from build123d import *

# Parameters (mm, degrees)
BOSS_EXTRUDE1_DEPTH = 300
SKETCH3_R           = 1.6
CUT_EXTRUDE1_DEPTH  = 331.850051567
CUT_EXTRUDE2_START  = -2
SKETCH4_R           = 2.875
CUT_EXTRUDE2_DEPTH  = 329.850051657


with BuildPart() as part:
    # Sketch2 → Boss-Extrude1 (new body)
    with BuildSketch(Plane.XY):
        with BuildLine():
            Line((-10, 0), (-10, 57.592991829))
            Line((-10, 57.592991829), (-14, 57.592991829))
            Line((-14, 57.592991829), (-14, 59.592991829))
            Line((-14, 59.592991829), (-10, 59.592991829))
            Line((-10, 59.592991829), (-5, 59.592991829))
            Line((-5, 59.592991829), (-5, 0))
            ThreePointArc((-5, 0), (-3.13691529, -11.76748288), (2.270101024, -22.383928263))
            Line((2.270101024, -22.383928263), (29.120915128, -37.886253013))
            ThreePointArc((29.120915128, -37.886253013), (41.018534684, -37.260643809), (52.141016151, -32.990381057))
            Line((52.141016151, -32.990381057), (103.750060963, -3.193885142))
            Line((103.750060963, -3.193885142), (106.250060963, -7.524012161))
            Line((106.250060963, -7.524012161), (108.250060963, -10.988113776))
            Line((108.250060963, -10.988113776), (106.518010155, -11.988113776))
            Line((106.518010155, -11.988113776), (104.518010155, -8.524012161))
            Line((104.518010155, -8.524012161), (54.641016151, -37.320508076))
            ThreePointArc((54.641016151, -37.320508076), (11.547005384, -37.320508076), (-10, 0))
        make_face()
    extrude(amount=BOSS_EXTRUDE1_DEPTH)

    # Sketch3 → Cut-Extrude1 (cut, through all)
    with BuildSketch(Plane(origin=(-9.125, -15.804963619, 0), x_dir=(0.8660254037844395, -0.49999999999999856, 0), z_dir=(0.49999999999999856, 0.8660254037844395, 0))):
        with Locations(Location((28.660254038, -15, 0), (0, 0, 180))):
            Circle(SKETCH3_R)
        with Locations(Location((28.660254038, -285, 0), (0, 0, 180))):
            Circle(SKETCH3_R)
    extrude(amount=-CUT_EXTRUDE1_DEPTH, mode=Mode.SUBTRACT)

    # Sketch4 → Cut-Extrude2 (cut, through all)
    with BuildSketch(Plane(origin=(-9.125, -15.804963619, 0), x_dir=(0.8660254037844395, -0.49999999999999856, 0), z_dir=(0.49999999999999856, 0.8660254037844395, 0)).offset(CUT_EXTRUDE2_START)):
        with Locations(Location((28.660254038, -15, 0), (0, 0, 180))):
            Circle(SKETCH4_R)
        with Locations(Location((28.660254038, -285, 0), (0, 0, 180))):
            Circle(SKETCH4_R)
    extrude(amount=-CUT_EXTRUDE2_DEPTH, mode=Mode.SUBTRACT)


solid = part.part
Geometry check sheet. Reference: the model listing, model coordinates, mm. A direction names the side the tool comes from. Coordinates: 2 decimals unless noted, no trailing zeros. Loops run counter-clockwise (first coordinate to the right, second up) from the corner with the lowest first, then second, coordinate; pieces in that order, holes last. Notation, with made-up numbers: (60, -26) - (105, -26) arc R18 ccw to (105, -3) - close; hole circle Ø2 at (20.25, -17.75). An arc over 180 degrees is marked (long way). Use one line per item in the form item = value. Start each with the question number.
Item 1: Tool access check on faces 1 (the face through (13.47, -34.74, 287.85)), 2 (the face through (15.51, -30.03, 147.9)), 3 (the face through (-10, 28, 148)). Record the directions out of +Z, -Z, +X, -X, +Y, -Y that give a thin tool (end or side, any length) a straight path to the whole face; none if there is none.
Item 2: Thickness scan on probe 1 along Y at (x, z) = (31, 179); probe 2 along X at (y, z) = (-2, 182); probe 3 along X at (y, z) = (-16.5, 276.5). Record the ranges inside material, lowest first.
Item 3: Section check B-B, the plane y = 5. Enter the section's corners in (x, z).
Item 4: Gauge pin test, flat ends, axial feed: pin 1 (1 mm diameter, centred on y = 36.5, z = 207.5, fed in from -X); pin 2 (10 mm diameter, centred on y = -21, z = 111.5, fed in from +X); pin 3 (1.5 mm diameter, centred on x = 5, z = 259.5, fed in from +Y). Record the tip position at first contact, or that the pin passes through.
Item 5: Section check C-C, the plane x = 34. Enter the section's corners in (y, z), and give its area (3 significant figures).
Item 6: Section check A-A, the plane z = 25. Enter the section's corners in (x, y).
Item 7: Mould release check, pull along X, two halves, no side actions. Record for faces 4 (the face through (-3.188, -11.608, 147.9)), 5 (the face through (12.096, -37.632, 147.9)), 6 (the face through (-5, 30, 148)), 7 (the face through (20, -33, 0)): +X half, -X half, draft (parallel to the pull), parting line (faces both ways), or undercut.
Computed:
q1.face_1 = none
q1.face_2 = +Z, -Z, +Y
q1.face_3 = +Z, -Z, -X, -Y
q2.probe_1 = -43.04 to -38.04
q2.probe_2 = -9.95 to -4.95
q2.probe_3 = -6.72 to -1.24, 80.7 to 90.7
q3.outline = (-10, 0) - (-5, 0) - (-5, 300) - (-10, 300) - close
q4.pin_1 = -10
q4.pin_2 = 91.57
q4.pin_3 = -23.53
q5.outline = (-43.08, 0) - (-38.08, 0) - (-38.08, 300) - (-43.08, 300) - close
q5.area = 1,500 mm2
q6.outline = (-14, 57.59) - (-10, 57.59) - (-10, 0) arc R43.09 ccw to (54.64, -37.32) - (104.52, -8.52) - (106.52, -11.99) - (108.25, -10.99) - (103.75, -3.19) - (52.14, -32.99) arc R38.09 cw to (29.12, -37.89) - (2.27, -22.38) arc R38.09 cw to (-5, 0) - (-5, 59.59) - (-14, 59.59) - close
q7.face_4 = undercut
q7.face_5 = parting line
q7.face_6 = +X half
q7.face_7 = draft
